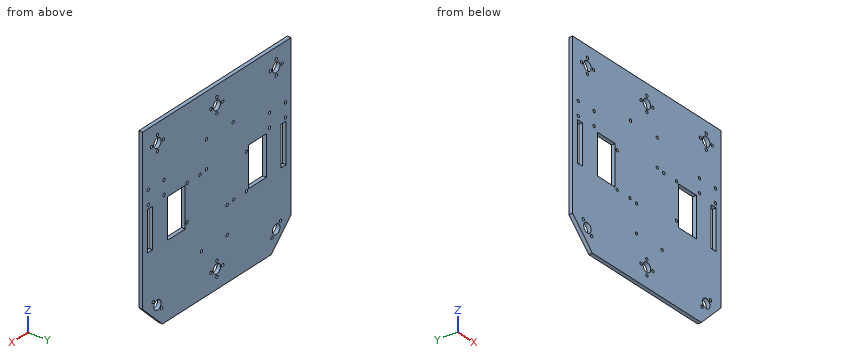
from build123d import *

# Parameters (mm, degrees)
ESQUISSE1_R              = 7.5
ESQUISSE1_R_2            = 2.3
ESQUISSE1_R_3            = 2.34
BOSS_EXTRU_1_DEPTH       = 6
ENL_V_MAT_EXTRU_9_DEPTH  = 10.5
ESQUISSE6_R              = 2.3
ENL_V_MAT_EXTRU_10_DEPTH = 50
ESQUISSE4_W              = 36
ESQUISSE4_H              = 64
ENL_V_MAT_EXTRU_11_DEPTH = 50
ESQUISSE11_R             = 2.3
ESQUISSE11_R_2           = 2.34
ENL_V_MAT_EXTRU_15_DEPTH = 10


with BuildPart() as part:
    # Esquisse1 → Boss.-Extru.1 (new body)
    with BuildSketch(Plane(origin=(0, 0, 0), x_dir=(1, 0, 0), z_dir=(0, 1, 0))):
        Polygon((-150, 0), (-150, 260), (-110, 300), (110, 300), (150, 260), (150, 0), align=None)
        with Locations(Location((-120, 30, 0), (0, 0, 270))):
            Circle(ESQUISSE1_R, mode=Mode.SUBTRACT)
        with Locations(Location((-120, 267.5, 0), (0, 0, 270))):
            Circle(ESQUISSE1_R, mode=Mode.SUBTRACT)
        with Locations(Location((120, 267.5, 0), (0, 0, 270))):
            Circle(ESQUISSE1_R, mode=Mode.SUBTRACT)
        with Locations(Location((-111.514718626, 275.985281374, 0), (0, 0, 270))):
            Circle(ESQUISSE1_R_2, mode=Mode.SUBTRACT)
        with Locations(Location((-128.485281374, 259.014718626, 0), (0, 0, 270))):
            Circle(ESQUISSE1_R_2, mode=Mode.SUBTRACT)
        with Locations(Location((111.514718626, 275.985281374, 0), (0, 0, 270))):
            Circle(ESQUISSE1_R_2, mode=Mode.SUBTRACT)
        with Locations(Location((128.485281374, 259.014718626, 0), (0, 0, 270))):
            Circle(ESQUISSE1_R_2, mode=Mode.SUBTRACT)
        with Locations(Location((120, 30, 0), (0, 0, 270))):
            Circle(ESQUISSE1_R, mode=Mode.SUBTRACT)
        with Locations(Location((120, 42, 0), (0, 0, 270))):
            Circle(ESQUISSE1_R_2, mode=Mode.SUBTRACT)
        with Locations(Location((-120, 42, 0), (0, 0, 270))):
            Circle(ESQUISSE1_R_2, mode=Mode.SUBTRACT)
        with Locations(Location((-120, 18, 0), (0, 0, 270))):
            Circle(ESQUISSE1_R_2, mode=Mode.SUBTRACT)
        with Locations(Location((-132, 30, 0), (0, 0, 270))):
            Circle(ESQUISSE1_R_2, mode=Mode.SUBTRACT)
        with Locations(Location((-108, 30, 0), (0, 0, 270))):
            Circle(ESQUISSE1_R_2, mode=Mode.SUBTRACT)
        with Locations(Location((108, 30, 0), (0, 0, 270))):
            Circle(ESQUISSE1_R_2, mode=Mode.SUBTRACT)
        with Locations(Location((132, 30, 0), (0, 0, 270))):
            Circle(ESQUISSE1_R_2, mode=Mode.SUBTRACT)
        with Locations(Location((120, 18, 0), (0, 0, 270))):
            Circle(ESQUISSE1_R_2, mode=Mode.SUBTRACT)
        with Locations(Location((0, 30, 0), (0, 0, 270))):
            Circle(ESQUISSE1_R, mode=Mode.SUBTRACT)
        with Locations(Location((0, 18, 0), (0, 0, 270))):
            Circle(ESQUISSE1_R_2, mode=Mode.SUBTRACT)
        with Locations(Location((12, 30, 0), (0, 0, 270))):
            Circle(ESQUISSE1_R_2, mode=Mode.SUBTRACT)
        with Locations(Location((0, 42, 0), (0, 0, 270))):
            Circle(ESQUISSE1_R_2, mode=Mode.SUBTRACT)
        with Locations(Location((-12, 30, 0), (0, 0, 270))):
            Circle(ESQUISSE1_R_2, mode=Mode.SUBTRACT)
        with Locations(Location((0, 270, 0), (0, 0, 270))):
            Circle(ESQUISSE1_R, mode=Mode.SUBTRACT)
        with Locations(Location((-12, 270, 0), (0, 0, 270))):
            Circle(ESQUISSE1_R_2, mode=Mode.SUBTRACT)
        with Locations(Location((0, 282, 0), (0, 0, 270))):
            Circle(ESQUISSE1_R_2, mode=Mode.SUBTRACT)
        with Locations(Location((12, 270, 0), (0, 0, 270))):
            Circle(ESQUISSE1_R_3, mode=Mode.SUBTRACT)
        with Locations(Location((0, 258, 0), (0, 0, 270))):
            Circle(ESQUISSE1_R_2, mode=Mode.SUBTRACT)
    extrude(amount=BOSS_EXTRU_1_DEPTH)

    # Esquisse7 → Enlèv. mat.-Extru.9 (cut)
    with BuildSketch(Plane(origin=(0, 6, 0), x_dir=(1, 0, 0), z_dir=(0, 1, 0))):
        Polygon((-130, 150), (-130, 182), (-140, 182), (-140, 118), (-130, 118), align=None)
    enl_v_mat_extru_9 = extrude(amount=-ENL_V_MAT_EXTRU_9_DEPTH, mode=Mode.SUBTRACT)

    # Esquisse6 → Enlèv. mat.-Extru.10 (cut)
    with BuildSketch(Plane(origin=(0, 6, 0), x_dir=(1, 0, 0), z_dir=(0, 1, 0))):
        with Locations(Location((-138.5, 90, 0), (0, 0, 270))):
            Circle(ESQUISSE6_R)
        with Locations(Location((-138.5, 112, 0), (0, 0, 270))):
            Circle(ESQUISSE6_R)
        with Locations(Location((-106.5, 112, 0), (0, 0, 270))):
            Circle(ESQUISSE6_R)
        with Locations(Location((-106.5, 90, 0), (0, 0, 270))):
            Circle(ESQUISSE6_R)
    enl_v_mat_extru_10 = extrude(amount=-ENL_V_MAT_EXTRU_10_DEPTH, mode=Mode.SUBTRACT)

    # Esquisse4 → Enlèv. mat.-Extru.11 (cut)
    with BuildSketch(Plane(origin=(0, 6, 0), x_dir=(1, 0, 0), z_dir=(0, 1, 0))):
        with Locations((-82, 150)):
            Rectangle(ESQUISSE4_W, ESQUISSE4_H)
    enl_v_mat_extru_11 = extrude(amount=-ENL_V_MAT_EXTRU_11_DEPTH, mode=Mode.SUBTRACT)

    # Symétrie1: Enlèv. mat.-Extru.9 across plane
    add(enl_v_mat_extru_9.mirror(Plane(origin=(0, 0, 0), x_dir=(0, 0, 1), z_dir=(1, 0, 0))), mode=Mode.SUBTRACT)

    # Symétrie2: Enlèv. mat.-Extru.11 across plane
    add(enl_v_mat_extru_11.mirror(Plane(origin=(0, 0, 0), x_dir=(0, 0, 1), z_dir=(1, 0, 0))), mode=Mode.SUBTRACT)

    # Symétrie3: Enlèv. mat.-Extru.10 across plane
    add(enl_v_mat_extru_10.mirror(Plane(origin=(0, 0, 0), x_dir=(0, 0, 1), z_dir=(1, 0, 0))), mode=Mode.SUBTRACT)

    # Esquisse11 → Enlèv. mat.-Extru.15 (cut)
    with BuildSketch(Plane(origin=(0, 6, 0), x_dir=(1, 0, 0), z_dir=(0, 1, 0))):
        with Locations(Location((34, 116, 0), (0, 0, 270))):
            Circle(ESQUISSE11_R)
        with Locations(Location((60, 116, 0), (0, 0, 270))):
            Circle(ESQUISSE11_R)
        with Locations(Location((60, 174, 0), (0, 0, 270))):
            Circle(ESQUISSE11_R)
        with Locations(Location((-21, 230, 0), (0, 0, 270))):
            Circle(ESQUISSE11_R)
        with Locations(Location((-21, 186, 0), (0, 0, 270))):
            Circle(ESQUISSE11_R)
        with Locations(Location((31, 230, 0), (0, 0, 270))):
            Circle(ESQUISSE11_R)
        with Locations(Location((-60, 126, 0), (0, 0, 270))):
            Circle(ESQUISSE11_R)
        with Locations(Location((-34, 184, 0), (0, 0, 270))):
            Circle(ESQUISSE11_R)
        with Locations(Location((-60, 184, 0), (0, 0, 270))):
            Circle(ESQUISSE11_R)
        with Locations(Location((-33, 70, 0), (0, 0, 270))):
            Circle(ESQUISSE11_R_2)
        with Locations(Location((21, 70, 0), (0, 0, 270))):
            Circle(ESQUISSE11_R)
        with Locations(Location((21, 114, 0), (0, 0, 270))):
            Circle(ESQUISSE11_R)
    extrude(amount=-ENL_V_MAT_EXTRU_15_DEPTH, mode=Mode.SUBTRACT)


solid = part.part
Read the model definition and answer for the solid it produces. Units are mm, in the model's axes. Give positions to 0.01 mm unless a question says otherwise; leave off trailing zeros. Loops run counter-clockwise (first coordinate to the right, second up) from the corner with the lowest first, then second, coordinate; pieces in that order, holes last. Notation, with made-up numbers: M 84.25,85.25 L 142.25,85.25 A19 ccw 142.25,118.25 Z; hole C 21.25,-6 d11. An arc over 180 degrees is marked long. Write each question's results on one line, items separated by ' | '.
1. Given pin 1 (3.5 mm diameter, centred on x = -12, z = -30, fed in from -Y), flat-ended and moving along its own axis, determine where the tip first touches the part or whether it passes through.
Values:
pin 1: passes through
2. Section B-B on y = 1.7 is taken. State how many separate pieces and enclosed holes the cut face has, plus the area to 3 significant figures.
Values:
separate pieces: 1 | enclosed holes: 50 | area: 80,800 mm^2
3. Straight lines are drawn through the part: line 1 (X direction, y = 4.5, z = -42); line 2 (X direction, y = 1.5, z = -70); line 3 (X direction, y = 0.35, z = -153). For each, find the intervals that lie inside material, in ascending order. Write a range as [from, to].
Values:
line 1: x = [-150, -122.3], [-117.7, -2.3], [2.3, 117.7], [122.3, 150] | line 2: x = [-150, -35.34], [-30.66, 18.7], [23.3, 150] | line 3: x = [-150, -140], [-130, -100], [-64, 64], [100, 130], [140, 150]
4. Section A-A on x = 74 is taken. Give the vertices of the cut face in (y, z).
Values:
outline: M 0,-300 L 6,-300 L 6,-182 L 0,-182 Z; M 0,-118 L 6,-118 L 6,0 L 0,0 Z
